Here's the drawing with two shaded views (mm, measured from the low corner). I have some questions. A direction names the side the tool comes from. Give positions to 0.01 mm unless a question says otherwise; leave off trailing zeros. Loops run counter-clockwise (first coordinate to the right, second up) from the corner with the lowest first, then second, coordinate; pieces in that order, holes last. Notation, with made-up numbers: M 10,-33.5 L 57,-33.5 A13 cw 57,-18.5 Z; hole C 79,68.25 d4. An arc over 180 degrees is marked long. Put each result on its own line as item: value. Start each with the question number.
1) Imagine slicing it at C-C (y = 48). Write out the boundary of the cut face in (x, z), then the cut area to 3 significant figures.
2) Imagine slicing it at A-A (z = 3). Write out the boundary of the cut face in (x, y), then the cut area to 3 significant figures.
3) If we mould it in two halves opening along X, with no side actions, what happens to the marked faces 6, 7 and 8? For each: +X half, -X half, draft (parallel to the pull), parting line (faces both ways), or undercut.
4) For the marked faces 1, 2, 3, 4 and 5, which set-ups out of +Z, -Z, +X, -X, +Y, -Y let a thin tool reach every point of the face, with its end or its side?
5) Imagine slicing it at D-D (x = 27.5). Write out the boundary of the cut face in (y, z), then the cut area to 3 significant figures.
6) For P1, Ø2, axis at x = 57.5, z = 27, coming from the -Y side; P2, Ø8, axis at x = 29.5, z = 16, coming from the -Y side; P3, Ø7.5, axis at y = 54, z = 16.5, coming from the -X side, each with a flat end and sliding along its axis, tell me the tip position at first contact or that it passes through.
7) Imagine slicing it at B-B (y = 6.5). Write out the boundary of the cut face in (x, z).
8) Please list where these lines run through material, in increasing order: line 1 along X through (y, z) = (3, 9) (1 decimal); line 2 along X through (y, z) = (59.5, 12); line 3 along X through (y, z) = (5.5, 8.5) (1 decimal). Write a range as from..to.
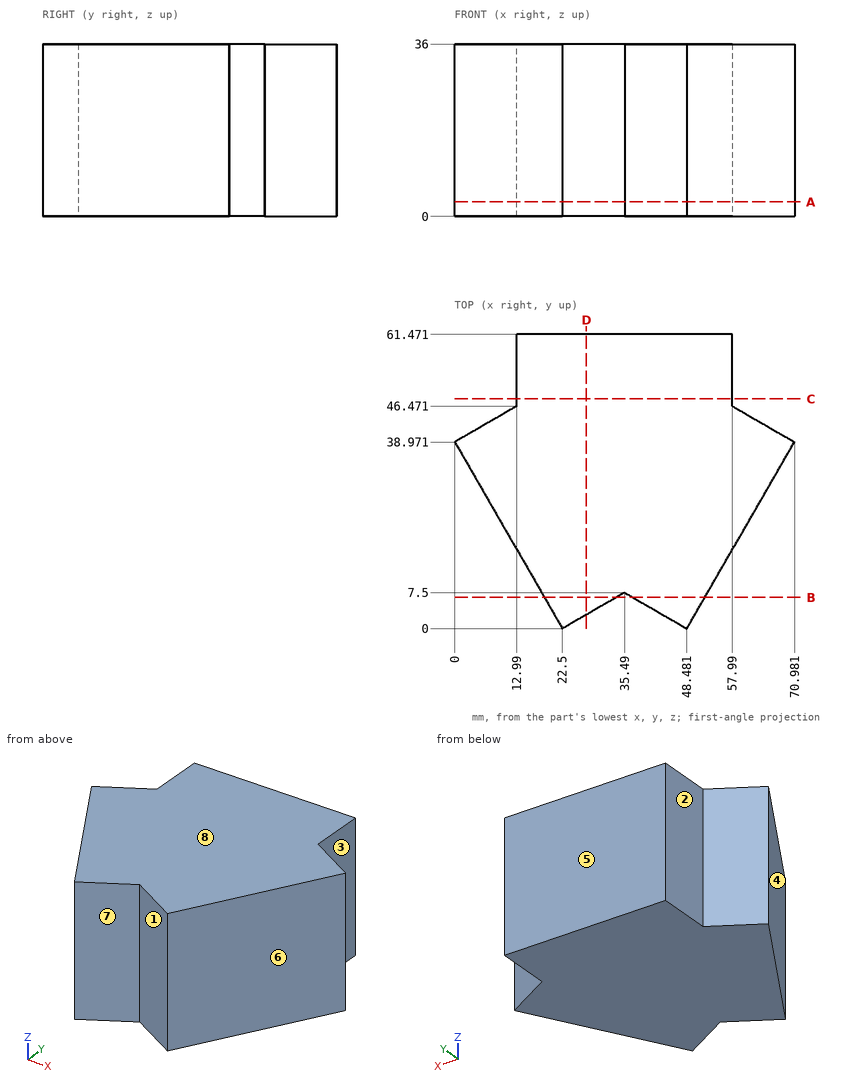
Recorded:
1. outline: M 12.99,0 L 57.99,0 L 57.99,36 L 12.99,36 Z
1. area: 1,620 mm²
2. outline: M 0,38.97 L 22.5,0 L 35.49,7.5 L 48.48,0 L 70.98,38.97 L 57.99,46.47 L 57.99,61.47 L 12.99,61.47 L 12.99,46.47 Z
2. area: 2,900 mm²
3. face 6: +X half
3. face 7: undercut
3. face 8: draft
4. face 1: +Z, -Z, -Y
4. face 2: +Z, -Z, -X, +Y
4. face 3: +Z, -Z, +X, +Y
4. face 4: +Z, -Z, -X, -Y
4. face 5: +Z, -Z, +X, -X, +Y
5. outline: M 2.89,0 L 61.47,0 L 61.47,36 L 2.89,36 Z
5. area: 2,110 mm²
6. P1: y = 13.89
6. P2: y = 1.73
6. P3: x = 12.99
7. outline: M 18.75,0 L 33.76,0 L 33.76,36 L 18.75,36 Z; M 37.22,0 L 52.23,0 L 52.23,36 L 37.22,36 Z
8. line 1: 20.8..27.7, 43.3..50.2
8. line 2: 12.99..57.99
8. line 3: 19.3..32, 39..51.7
